Verification items for this drawing (mm, ordinates from the low corner). Coordinates: 2 decimals unless noted, no trailing zeros. Order: outer loops, then holes, each group sorted by start corner. A loop starts at its lowest first (then second) coordinate and runs counter-clockwise, first axis right, second up. Notation, with made-up numbers: M -28.75,66.25 L -7.75,66.25 A20 cw -7.75,96.25 Z; hole C 77.25,33.5 d2. An arc over 180 degrees is marked long. Return JSON: item names as keys, results as strings. Group by question number.
1. Section check A-A, the plane z = 90. Record the cut outline in (x, y).
2. Material ranges on line 1 along X through (y, z) = (1.3, 10); line 2 along X through (y, z) = (2.8, 89), recorded low to high.
3. Gauge pin test, flat end, axial feed: pin 1 (1.5 mm diameter, centred on x = 48, y = 1, fed in from -Z). Record the tip position at first contact, or that the pin passes through.
4. Section check B-B, the plane x = 10. Record the cut outline in (y, z), plus the area to 3 significant figures.
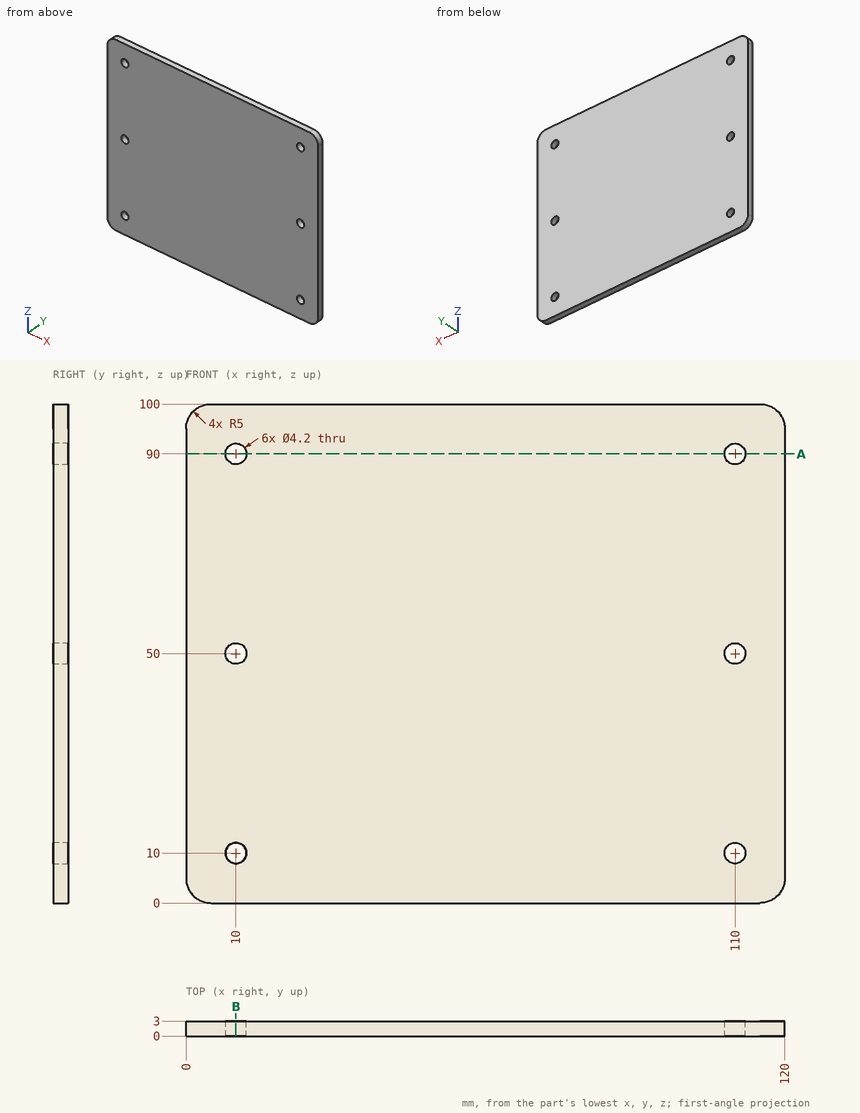
Answers follow:
{
 "1": {"outline": "M 0,0 L 7.9,0 L 7.9,3 L 0,3 Z; M 12.1,0 L 107.9,0 L 107.9,3 L 12.1,3 Z; M 112.1,0 L 120,0 L 120,3 L 112.1,3 Z"},
 "2": {"line 1": "0 to 7.9, 12.1 to 107.9, 112.1 to 120", "line 2": "0 to 8.15, 11.85 to 108.15, 111.85 to 120"},
 "3": {"pin 1": "z = 0"},
 "4": {"outline": "M 0,0 L 3,0 L 3,7.9 L 0,7.9 Z; M 0,12.1 L 3,12.1 L 3,47.9 L 0,47.9 Z; M 0,52.1 L 3,52.1 L 3,87.9 L 0,87.9 Z; M 0,92.1 L 3,92.1 L 3,100 L 0,100 Z", "area": "262 mm^2"}
}
